CAD build for the part. Positions are in the model's coordinates, mm. Round coordinates to 2 decimals unless told otherwise and drop trailing zeros. Loops run counter-clockwise (first coordinate to the right, second up) from the corner with the lowest first, then second, coordinate; pieces in that order, holes last. Notation, with made-up numbers: M -8.75,70.5 L 5.25,70.5 A15 ccw 5.25,94.5 Z; hole C 35,-12 d5. An arc over 180 degrees is marked long. Use one line per item in the form item = value.
from build123d import *

# Parameters (mm, degrees)
SKETCH1_W           = 170.67
SKETCH1_H           = 92.67
BOSS_EXTRUDE3_DEPTH = 10


with BuildPart() as part:
    # Sketch1 → Boss-Extrude3 (new body)
    with BuildSketch(Plane.XY):
        with Locations((49.728369838, 28.496112047)):
            Rectangle(SKETCH1_W, SKETCH1_H)
        Polygon((-22.271785995, -14.851567408), (-22.271785995, -2.851567408), (-22.334139111, -2.851567408), (-22.334139111, 9.148432592), (-9.334139111, 9.148432592), (-9.334139111, -2.851567408), (-9.271785995, -2.851567408), (-9.271785995, -14.851567408), align=None, mode=Mode.SUBTRACT)
        Polygon((-2.896492227, -14.851567408), (-2.896492227, -2.851567408), (-2.834139111, -2.851567408), (-2.834139111, 9.148432592), (10.165860889, 9.148432592), (10.165860889, -2.851567408), (10.103507773, -2.851567408), (10.103507773, -14.851567408), align=None, mode=Mode.SUBTRACT)
        Polygon((16.665860889, -2.851567408), (16.665860889, 9.148432592), (29.665860889, 9.148432592), (29.665860889, -2.851567408), (29.728214005, -2.851567408), (29.728214005, -14.851567408), (16.728214005, -14.851567408), (16.728214005, -2.851567408), align=None, mode=Mode.SUBTRACT)
        Polygon((36.165860889, -2.851567408), (36.165860889, 9.148432592), (49.165860889, 9.148432592), (49.165860889, -2.851567408), (49.228214005, -2.851567408), (49.228214005, -14.851567408), (36.228214005, -14.851567408), (36.228214005, -2.851567408), align=None, mode=Mode.SUBTRACT)
        Polygon((-9.334139111, 27.148432592), (-9.334139111, 15.148432592), (-22.334139111, 15.148432592), (-22.334139111, 27.148432592), (-22.396492227, 27.148432592), (-22.396492227, 39.148432592), (-9.396492227, 39.148432592), (-9.396492227, 27.148432592), align=None, mode=Mode.SUBTRACT)
        Polygon((10.165860889, 27.148432592), (10.165860889, 15.148432592), (-2.834139111, 15.148432592), (-2.834139111, 27.148432592), (-2.896492227, 27.148432592), (-2.896492227, 39.148432592), (10.103507773, 39.148432592), (10.103507773, 27.148432592), align=None, mode=Mode.SUBTRACT)
        Polygon((29.728214005, 39.148432592), (29.728214005, 27.148432592), (29.665860889, 27.148432592), (29.665860889, 15.148432592), (16.665860889, 15.148432592), (16.665860889, 27.148432592), (16.728214005, 27.148432592), (16.728214005, 39.148432592), align=None, mode=Mode.SUBTRACT)
        Polygon((49.228214005, 39.148432592), (49.228214005, 27.148432592), (49.165860889, 27.148432592), (49.165860889, 15.148432592), (36.165860889, 15.148432592), (36.165860889, 27.148432592), (36.228214005, 27.148432592), (36.228214005, 39.148432592), align=None, mode=Mode.SUBTRACT)
        Polygon((55.665860889, 9.148432592), (68.665860889, 9.148432592), (68.665860889, -2.851567408), (68.728214005, -2.851567408), (68.728214005, -14.851567408), (55.728214005, -14.851567408), (55.728214005, -2.851567408), (55.665860889, -2.851567408), align=None, mode=Mode.SUBTRACT)
        Polygon((75.165860889, 9.148432592), (88.165860889, 9.148432592), (88.165860889, -2.851567408), (88.228214005, -2.851567408), (88.228214005, -14.851567408), (75.228214005, -14.851567408), (75.228214005, -2.851567408), (75.165860889, -2.851567408), align=None, mode=Mode.SUBTRACT)
        Polygon((94.603507773, -14.851567408), (94.603507773, -2.851567408), (94.665860889, -2.851567408), (94.665860889, 9.148432592), (107.665860889, 9.148432592), (107.665860889, -2.851567408), (107.603507773, -2.851567408), (107.603507773, -14.851567408), align=None, mode=Mode.SUBTRACT)
        Polygon((127.165860889, -2.851567408), (127.103507773, -2.851567408), (127.103507773, -14.851567408), (114.103507773, -14.851567408), (114.103507773, -2.851567408), (114.165860889, -2.851567408), (114.165860889, 9.148432592), (127.165860889, 9.148432592), align=None, mode=Mode.SUBTRACT)
        Polygon((68.728214005, 39.148432592), (68.728214005, 27.148432592), (68.665860889, 27.148432592), (68.665860889, 15.148432592), (55.665860889, 15.148432592), (55.665860889, 27.148432592), (55.728214005, 27.148432592), (55.728214005, 39.148432592), align=None, mode=Mode.SUBTRACT)
        Polygon((88.228214005, 39.148432592), (88.228214005, 27.148432592), (88.165860889, 27.148432592), (88.165860889, 15.148432592), (75.165860889, 15.148432592), (75.165860889, 27.148432592), (75.228214005, 27.148432592), (75.228214005, 39.148432592), align=None, mode=Mode.SUBTRACT)
        Polygon((94.665860889, 27.148432592), (94.728214005, 27.148432592), (94.728214005, 39.148432592), (107.728214005, 39.148432592), (107.728214005, 27.148432592), (107.665860889, 27.148432592), (107.665860889, 15.148432592), (94.665860889, 15.148432592), align=None, mode=Mode.SUBTRACT)
        Polygon((127.228214005, 39.148432592), (127.228214005, 27.148432592), (127.165860889, 27.148432592), (127.165860889, 15.148432592), (114.165860889, 15.148432592), (114.165860889, 27.148432592), (114.228214005, 27.148432592), (114.228214005, 39.148432592), align=None, mode=Mode.SUBTRACT)
        Polygon((-22.396492227, 44.753067208), (-22.396492227, 56.753067208), (-22.334139111, 56.753067208), (-22.334139111, 68.753067208), (-9.334139111, 68.753067208), (-9.334139111, 56.753067208), (-9.396492227, 56.753067208), (-9.396492227, 44.753067208), align=None, mode=Mode.SUBTRACT)
        Polygon((10.165860889, 56.753067208), (10.103507773, 56.753067208), (10.103507773, 44.753067208), (-2.896492227, 44.753067208), (-2.896492227, 56.753067208), (-2.834139111, 56.753067208), (-2.834139111, 68.753067208), (10.165860889, 68.753067208), align=None, mode=Mode.SUBTRACT)
        Polygon((16.603507773, 44.753067208), (16.603507773, 56.753067208), (16.665860889, 56.753067208), (16.665860889, 68.753067208), (29.665860889, 68.753067208), (29.665860889, 56.753067208), (29.603507773, 56.753067208), (29.603507773, 44.753067208), align=None, mode=Mode.SUBTRACT)
        Polygon((36.103507773, 44.753067208), (36.103507773, 56.753067208), (36.165860889, 56.753067208), (36.165860889, 68.753067208), (49.165860889, 68.753067208), (49.165860889, 56.753067208), (49.103507773, 56.753067208), (49.103507773, 44.753067208), align=None, mode=Mode.SUBTRACT)
        Polygon((55.665860889, 68.753067208), (68.665860889, 68.753067208), (68.665860889, 56.753067208), (68.728214005, 56.753067208), (68.728214005, 44.753067208), (55.728214005, 44.753067208), (55.728214005, 56.753067208), (55.665860889, 56.753067208), align=None, mode=Mode.SUBTRACT)
        Polygon((75.165860889, 68.753067208), (88.165860889, 68.753067208), (88.165860889, 56.753067208), (88.228214005, 56.753067208), (88.228214005, 44.753067208), (75.228214005, 44.753067208), (75.228214005, 56.753067208), (75.165860889, 56.753067208), align=None, mode=Mode.SUBTRACT)
        Polygon((94.665860889, 68.753067208), (107.665860889, 68.753067208), (107.665860889, 56.753067208), (107.728214005, 56.753067208), (107.728214005, 44.753067208), (94.728214005, 44.753067208), (94.728214005, 56.753067208), (94.665860889, 56.753067208), align=None, mode=Mode.SUBTRACT)
        Polygon((114.165860889, 56.753067208), (114.165860889, 68.753067208), (127.165860889, 68.753067208), (127.165860889, 56.753067208), (127.228214005, 56.753067208), (127.228214005, 44.753067208), (114.228214005, 44.753067208), (114.228214005, 56.753067208), align=None, mode=Mode.SUBTRACT)
    extrude(amount=BOSS_EXTRUDE3_DEPTH)


solid = part.part
1. Cut at A-A on x = -20. Write the cut outline in (y, z).
Completed:
outline = M -17.84,0 L -14.85,0 L -14.85,10 L -17.84,10 Z; M 9.15,0 L 15.15,0 L 15.15,10 L 9.15,10 Z; M 39.15,0 L 44.75,0 L 44.75,10 L 39.15,10 Z; M 68.75,0 L 74.83,0 L 74.83,10 L 68.75,10 Z
2. Probe line 1 along Y through (x, z) = (23, 3.75). List the from-to ranges inside material, lowest first. Write a range as from..to.
Completed:
line_1 = -17.84..-14.85, 9.15..15.15, 39.15..44.75, 68.75..74.83
3. Cut at B-B on z = 5. State how many separate pieces and enclosed holes the cut face has, and give its area (3 significant figures).
Completed:
separate_pieces = 1
enclosed_holes = 24
area = 8,330 mm2
4. Pull direction Y, two halves, no side cores. Call faces 1 (the face through (121, 68.753, 5)), 2 (the face through (49, -17.839, 5)), 3 (the face through (11, 39, 10)): +Y half, -Y half, draft (parallel to the pull), parting line (faces both ways), or undercut.
Completed:
face_1 = undercut
face_2 = -Y half
face_3 = draft
